from build123d import *

# Parameters (mm, degrees)
SKETCH1_W           = 1520
SKETCH1_H           = 20
BASE_FLANGE1_DEPTH  = 2.5
SKETCH6_R           = 3.5
CUT_EXTRUDE1_DEPTH  = 10
LPATTERN1_COUNT     = 6
LPATTERN1_PITCH     = 146
LPATTERN1_COL_COUNT = 6
LPATTERN1_COL_PITCH = 146


# Sheet-metal steps are written as plain solids
with BuildPart() as part:
    # Sketch1 → Base-Flange1 (new body)
    with BuildSketch(Plane(origin=(0, 0, 0), x_dir=(1, 0, 0), z_dir=(0, 1, 0))):
        Rectangle(SKETCH1_W, SKETCH1_H)
    extrude(amount=-BASE_FLANGE1_DEPTH)

    # Sketch6 → Cut-Extrude1 (cut)
    with BuildSketch(Plane(origin=(0, 0, 0), x_dir=(1, 0, 0), z_dir=(0, 1, 0))):
        with Locations(Location((0, 0, 0), (0, 0, 270))):
            Circle(SKETCH6_R)
    cut_extrude1 = extrude(amount=-CUT_EXTRUDE1_DEPTH, mode=Mode.SUBTRACT)

    # LPattern1: Cut-Extrude1 ×6
    with Locations(*[(-i * LPATTERN1_PITCH, 0, 0) for i in range(1, LPATTERN1_COUNT)]):
        add(cut_extrude1, mode=Mode.SUBTRACT)

    # LPattern1 col: Cut-Extrude1 ×6
    with Locations(*[(i * LPATTERN1_COL_PITCH, 0, 0) for i in range(1, LPATTERN1_COL_COUNT)]):
        add(cut_extrude1, mode=Mode.SUBTRACT)


solid = part.part
Here's how the part is built. I have some questions about the finished solid (model axes, mm). Round coordinates to 2 decimals unless told otherwise and drop trailing zeros. Return JSON: item names as keys, results as strings. Group by question number.
1. If we section it at A-A on z = 0: State how many separate pieces and enclosed holes the cut face has, then the cut area to 3 significant figures.
2. I'm going to push a flat-ended pin straight in: pin 1 Ø11 at (x, z) = (584, 0) entering from -Y. Where does the tip first touch, or does it pass through?
3. Please list where these lines run through material, in increasing order: probe 1 along Z at (x, y) = (-292, -0.45); probe 2 along Z at (x, y) = (-440, -0.75).
Reply:
{
 "1": {"separate pieces": "12", "enclosed holes": "0", "area": "3,610 mm^2"},
 "2": {"pin 1": "y = -2.5"},
 "3": {"probe 1": "-10 to -3.5, 3.5 to 10", "probe 2": "-10 to -2.87, 2.87 to 10"}
}
